from build123d import *

# Parameters (mm, degrees)
EXTRUDE_365_DEPTH = 5.3
SKETCH_4_W        = 0.6
SKETCH_4_H        = 11.005553499
CHAMFER_2062_SIZE = 1
FILLET_2107_R     = 0.4


with BuildPart() as part:
    # 草图1 → Extrude 365 (new body)
    with BuildSketch(Plane(origin=(0, 0, 0), x_dir=(0, 0, -1), z_dir=(1, 0, 0))):
        Polygon((6.5, 3.75277675), (6.5, -3.75277675), (0, -7.505553499), (-6.5, -3.75277675), (-6.5, 3.75277675), (0, 7.505553499), align=None)
    extrude(amount=EXTRUDE_365_DEPTH)

    # 草图2 → 凸台-旋转1 (revolve)
    with BuildSketch(Plane.XY, mode=Mode.PRIVATE) as revolve_1_sk:
        Polygon((0, 0), (70.3, 0), (70.3, 2.9175), (70.3, 4), (7.791693541, 4), (0, 4), align=None)
    revolve(revolve_1_sk.sketch.rotate(Axis((0, 0, 0), (1, 0, 0)), 90), axis=Axis((0, 0, 0), (1, 0, 0)))

    # 草图3 → 切除-旋转1 (revolve, cut)
    with BuildSketch(Plane.XY):
        Polygon((0, 6.5), (3.46730793, 12.505553499), (3.46730793, 17.505553499), (-10, 17.505553499), (-10, 6.5), align=None)
    revolve(axis=Axis((0, 0, 0), (1, 0, 0)), mode=Mode.SUBTRACT)

    # 草图5 → 切除-旋转2 (revolve, cut)
    with BuildSketch(Plane.XY):
        Polygon((5.3, 6.5), (1.83269207, 12.505553499), (1.83269207, 17.505553499), (11.83269207, 17.505553499), (11.83269207, 6.5), align=None)
    revolve(axis=Axis((0, 0, 0), (1, 0, 0)), mode=Mode.SUBTRACT)

    # 草图4 → 切除-旋转3 (revolve, cut)
    with BuildSketch(Plane.XY, mode=Mode.PRIVATE) as cut_revolve_3_sk:
        with Locations((5, 12.00277675)):
            Rectangle(SKETCH_4_W, SKETCH_4_H)
    revolve(cut_revolve_3_sk.sketch.rotate(Axis((0, 0, 0), (1, 0, 0)), 270), axis=Axis((0, 0, 0), (1, 0, 0)), mode=Mode.SUBTRACT)

    # Chamfer 2062
    chamfer_2062_edges = [part.edges().sort_by_distance(p)[0] for p in [
        (70.3, 0, -4),
    ]]
    chamfer(chamfer_2062_edges, length=CHAMFER_2062_SIZE)

    # Fillet 2107
    fillet_2107_edges = [part.edges().sort_by_distance(p)[0] for p in [
        (5.3, 0, -4),
    ]]
    fillet(fillet_2107_edges, radius=FILLET_2107_R)


solid = part.part
Here's how the part is built. I have some questions about the finished solid (model axes, mm). A direction names the side the tool comes from. Give positions to 0.01 mm unless a question says otherwise; leave off trailing zeros. Order: outer loops, then holes, each group sorted by start corner. A loop starts at its lowest first (then second) coordinate and runs counter-clockwise, first axis right, second up. Notation, with made-up numbers: (15.5, 5) -> (32.5, 5) arc R21 cw to (32.5, 32) -> close; hole circle Ø9 at (-15.5, 76). An arc over 180 degrees is marked (long way). One line per item, written item: value. Start each with the question number.
1. Will these pins go through, and if not, where does the flat tip stop? pin 1 Ø2 at (y, z) = (-0.5, -4.5) entering from +X; pin 2 Ø1.6 at (y, z) = (-1.5, -5.5) entering from +X; pin 3 Ø6 at (x, z) = (9.5, 1.5) entering from +Y; pin 4 Ø2 at (y, z) = (3.5, -2.5) entering from -X.
2. Imagine slicing it at A-A, the plane x = 12. List the corners of the cut face in (y, z) for me.
3. For faces 1 (the face through (4.7, -3, -6)), 2 (the face through (4.7, 3, 6)), 3 (the face through (37.055, 3.905, -0.867)), which set-ups out of +Z, -Z, +X, -X, +Y, -Y let a thin tool reach every point of the face, with its end or its side?
4. I need wall thicknesses on probe 1 along X at (y, z) = (5.25, -3.5); probe 2 along Y at (x, z) = (18.5, 0); probe 3 along Y at (x, z) = (49, -2). Which ranges of each line are inside material? Lowest first, please. Write a range as from..to.
Values follow:
1. pin 1: stops at x = 69.77
1. pin 2: stops at x = 5.3
1. pin 3: stops at y = 4
1. pin 4: stops at x = 0
2. outline: circle Ø8 at (0, 0)
3. face 1: -Z, +X, -Y
3. face 2: +Z, +X, +Y
3. face 3: +X
4. probe 1: x = 0..5.3
4. probe 2: y = -4..4
4. probe 3: y = -3.46..3.46
